Build history of the part. All positions in model axes, mm. Give positions to 0.01 mm unless a question says otherwise; leave off trailing zeros. Write each loop counter-clockwise with the first axis right and the second up, starting at its lowest first coordinate (ties: lowest second). Pieces come first, ordered by that corner, then holes. Notation, with made-up numbers: (2.25, 59) -> (41.25, 59) arc R30 ccw to (41.25, 81) -> close; hole circle Ø3 at (53, 81.5). An arc over 180 degrees is marked (long way). Put each result on its own line as item: value. Start each with the question number.
Item 1: Slice it at D-D, the plane x = -51.5. List the corners of the cut face in (y, z), plus the area to 3 significant figures.
Item 2: Drill centre lines: line 1 along X through (y, z) = (-0.65, -18); line 2 along Z through (x, y) = (23, 0); line 3 along X through (y, z) = (4.5, 6.5). Where is each one in solid material? Low to high.
Item 3: Slice it at A-A, the plane x = 0. List the corners of the cut face in (y, z), plus the area to 3 significant figures.
Item 4: Slice it at C-C, the plane z = 0. List the corners of the cut face in (x, y).
Item 5: Flat gauge pins, fed straight in: pin 1 Ø4.5 at (x, y) = (-40.5, 0) entering from +Z; pin 2 Ø6 at (y, z) = (6.5, 19.5) entering from +X; pin 3 Ø20 at (x, z) = (-22, -16.5) entering from +Y; pin 4 Ø4 at (y, z) = (2.5, 18) entering from +X. Where does each tip first touch, or does it go through?
Item 6: Slice it at B-B, the plane y = 3. List the corners of the cut face in (x, z), plus the area to 3 significant figures.
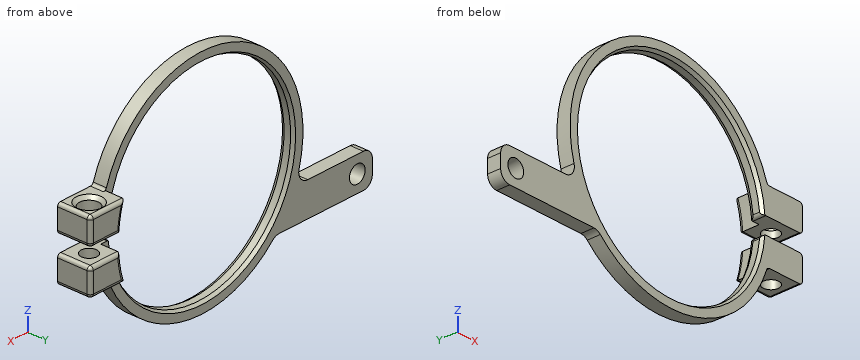
```python
from build123d import *

# Parameters (mm, degrees)
SKETCH_1_R          = 33.5
SKETCH_1_R_2        = 30.5
EXTRUDE_1_DEPTH     = 2
SKETCH_3_W          = 10
SKETCH_3_H          = 5
CUT_EXTRUDE_1_DEPTH = 48.544715795
EXTRUDE_START       = 10
EXTRUDE_2_DEPTH     = 10
SKETCH_5_R          = 2.9
CUT_EXTRUDE_2_DEPTH = 6
SKETCH_6_R          = 2.4
CUT_EXTRUDE_3_DEPTH = 59.242009954
FILLET_9_R          = 1
FILLET_11_R         = 1
FILLET_12_R         = 1
CHAMFER_1_SIZE      = 1
SKETCH_7_R          = 2.6
EXTRUDE_3_DEPTH     = 4
FILLET_13_R         = 3
CHAMFER_2_SIZE      = 1
CHAMFER_2_SIZE2     = 0.577350269
CHAMFER_3_SIZE      = 1
CHAMFER_3_SIZE2     = 0.577350269
FILLET_14_R         = 1


with BuildPart() as part:
    # 草圖1 → 填料-伸長1 (new, symmetric)
    with BuildSketch(Plane(origin=(0, 0, 0), x_dir=(1, 0, 0), z_dir=(0, 1, 0))):
        with Locations(Location((0, 0, 0), (0, 0, 270))):
            Circle(SKETCH_1_R)
        with Locations(Location((0, 0, 0), (0, 0, 270))):
            Circle(SKETCH_1_R_2, mode=Mode.SUBTRACT)
    extrude(amount=EXTRUDE_1_DEPTH, both=True)

    # 草圖3 → 除料-伸長1 (cut, through all)
    with BuildSketch(Plane(origin=(0, 2, 0), x_dir=(1, 0, 0), z_dir=(0, 1, 0))):
        with Locations((35.397368307, 0)):
            Rectangle(SKETCH_3_W, SKETCH_3_H)
    extrude(amount=-CUT_EXTRUDE_1_DEPTH, mode=Mode.SUBTRACT)

    # 草圖4 → 填料-伸長2 (add)
    with BuildSketch(Plane(origin=(0, -2, 0), x_dir=(1, 0, 0), z_dir=(0, 1, 0)).offset(EXTRUDE_START)):
        with BuildLine():
            Line((33.406586177, -2.5), (43.406586177, -2.5))
            Line((43.406586177, -2.5), (43.406586177, -10.5))
            Line((43.406586177, -10.5), (31.811947441, -10.5))
            ThreePointArc((31.811947441, -10.5), (32.853679883, -6.548718819), (33.406586177, -2.5))
        make_face()
        with BuildLine():
            Line((43.406586177, 10.5), (31.811947441, 10.5))
            ThreePointArc((31.811947441, 10.5), (32.853679883, 6.548718819), (33.406586177, 2.5))
            Line((33.406586177, 2.5), (43.406586177, 2.5))
            Line((43.406586177, 2.5), (43.406586177, 10.5))
        make_face()
    extrude(amount=-EXTRUDE_2_DEPTH)

    # 草圖5 → 除料-伸長2 (cut)
    with BuildSketch(Plane.XY.offset(10.5)):
        with Locations((38.406586177, 3)):
            Circle(SKETCH_5_R)
    extrude(amount=-CUT_EXTRUDE_2_DEPTH, mode=Mode.SUBTRACT)

    # 草圖6 → 除料-伸長3 (cut, through all)
    with BuildSketch(Plane.XY.offset(4.5)):
        with Locations((38.406586177, 3)):
            Circle(SKETCH_6_R)
    extrude(amount=-CUT_EXTRUDE_3_DEPTH, mode=Mode.SUBTRACT)

    # 圓角9
    fillet_9_edges = [part.edges().sort_by_distance(p)[0] for p in [
        (31.811947441, 0, 10.5),
        (31.811947441, 0, -10.5),
    ]]
    fillet(fillet_9_edges, radius=FILLET_9_R)

    # 圓角11
    fillet_11_edges = [part.edges().sort_by_distance(p)[0] for p in [
        (43.406586177, 3, 10.5),
        (43.406586177, 3, 2.5),
        (43.406586177, 3, -2.5),
        (43.406586177, 3, -10.5),
    ]]
    fillet(fillet_11_edges, radius=FILLET_11_R)

    # 圓角12
    fillet_12_edges = [part.edges().sort_by_distance(p)[0] for p in [
        (43.406586177, 8, -6.5),
        (43.113692958, 8, -2.792893219),
        (43.113692958, 8, -10.207106781),
        (37.906586177, 8, 2.5),
        (43.406586177, 8, 6.5),
        (43.113692958, 8, 10.207106781),
        (43.113692958, 8, 2.792893219),
        (32.853679883, 8, 6.548718819),
        (37.109266809, 8, 10.5),
        (32.853679883, 8, -6.548718819),
        (37.906586177, 8, -2.5),
        (37.109266809, 8, -10.5),
    ]]
    fillet(fillet_12_edges, radius=FILLET_12_R)

    # 導角1
    chamfer_1_edges = [part.edges().sort_by_distance(p)[0] for p in [
        (35.506586177, 3, 10.5),
    ]]
    chamfer(chamfer_1_edges, length=CHAMFER_1_SIZE)

    # 草圖7 → 填料-伸長3 (add)
    with BuildSketch(Plane(origin=(0, 2, 0), x_dir=(1, 0, 0), z_dir=(0, 1, 0))):
        with BuildLine():
            Line((-30.874746963, 13), (-56.5, 13))
            Line((-56.5, 13), (-56.5, 23))
            Line((-56.5, 23), (-24.356723918, 23))
            ThreePointArc((-24.356723918, 23), (-28.064725972, 18.292653064), (-30.874746963, 13))
        make_face()
        with Locations(Location((-51.5, 18, 0), (0, 0, 270))):
            Circle(SKETCH_7_R, mode=Mode.SUBTRACT)
    extrude(amount=-EXTRUDE_3_DEPTH)

    # 圓角13
    fillet_13_edges = [part.edges().sort_by_distance(p)[0] for p in [
        (-30.874746963, 0, -13),
        (-24.356723918, 0, -23),
        (-56.5, 0, -23),
        (-56.5, 0, -13),
    ]]
    fillet(fillet_13_edges, radius=FILLET_13_R)

    # 導角2
    chamfer_2_edges = [part.edges().sort_by_distance(p)[0] for p in [
        (-30.5, 2, 0),
    ]]
    chamfer_2_side = [part.faces().sort_by_distance(p)[0] for p in [
        (-30.5, 0, 0),
    ]]
    chamfer(chamfer_2_edges, length=CHAMFER_2_SIZE, length2=CHAMFER_2_SIZE2, reference=chamfer_2_side[0])

    # 導角3
    chamfer_3_edges = [part.edges().sort_by_distance(p)[0] for p in [
        (-30.5, -2, 0),
    ]]
    chamfer_3_side = [part.faces().sort_by_distance(p)[0] for p in [
        (-30.5, -0.5, 0),
    ]]
    chamfer(chamfer_3_edges, length=CHAMFER_3_SIZE, length2=CHAMFER_3_SIZE2, reference=chamfer_3_side[0])

    # 圓角14
    fillet_14_edges = [part.edges().sort_by_distance(p)[0] for p in [
        (30.397368307, 0, -2.5),
        (30.397368307, 0, 2.5),
    ]]
    fillet(fillet_14_edges, radius=FILLET_14_R)


solid = part.part
```
Values follow:
1. outline: (-2, -23) -> (2, -23) -> (2, -20.6) -> (-2, -20.6) -> close; (-2, -15.4) -> (2, -15.4) -> (2, -13) -> (-2, -13) -> close
1. area: 19.2 mm2
2. line 1: -56.5 to -54.1, -48.9 to -24.62, 24.62 to 28.25
2. line 2: -24.36 to -20.03, 20.03 to 24.36
2. line 3: 32.86 to 35.92, 40.89 to 43.41
3. outline: (-2, -33.5) -> (2, -33.5) -> (2, -31.08) -> (1, -30.5) -> (-1, -30.5) -> (-2, -31.08) -> close; (-2, 31.08) -> (-1, 30.5) -> (1, 30.5) -> (2, 31.08) -> (2, 33.5) -> (-2, 33.5) -> close
3. area: 22.8 mm2
4. outline: (-33.5, -2) -> (-31.08, -2) -> (-30.5, -1) -> (-30.5, 1) -> (-31.08, 2) -> (-33.5, 2) -> close
5. pin 1: z = -13
5. pin 2: through
5. pin 3: y = 2
5. pin 4: x = 29.4
6. outline: (31.81, -10.5) -> (36.01, -10.5) -> (36.01, -2.5) -> (33.41, -2.5) arc R33.5 cw to start; (31.81, 10.5) arc R33.5 cw to (33.41, 2.5) -> (36.01, 2.5) -> (36.01, 4.5) -> (35.51, 4.5) -> (35.51, 9.5) -> (34.51, 10.5) -> close; (40.81, -10.5) -> (42.41, -10.5) arc R1 ccw to (43.41, -9.5) -> (43.41, -3.5) arc R1 ccw to (42.41, -2.5) -> (40.81, -2.5) -> close; (40.81, 2.5) -> (42.41, 2.5) arc R1 ccw to (43.41, 3.5) -> (43.41, 9.5) arc R1 ccw to (42.41, 10.5) -> (42.31, 10.5) -> (41.31, 9.5) -> (41.31, 4.5) -> (40.81, 4.5) -> close
6. area: 85.4 mm2
